```python
from build123d import *

# Parameters (mm, degrees)
F0_W     = 108.2
F0_H     = 88.2
F0_W_2   = 105
F0_H_2   = 85
F1_DEPTH = 80
F2_W     = 108.2
F2_H     = 88.2
F2_W_2   = 105
F2_H_2   = 85
F3_DEPTH = 2
F4_R     = 2


with BuildPart() as f1:
    # F0 (on Top) → F1 (new body)
    with BuildSketch(Plane.XY):
        with Locations((52.5, 42.5)):
            Rectangle(F0_W, F0_H)
        with Locations((52.5, 42.5)):
            Rectangle(F0_W_2, F0_H_2, mode=Mode.SUBTRACT)
    extrude(amount=F1_DEPTH)

    # F2 (on face) → F3 (join)
    with BuildSketch(Plane(origin=(0, 0, 0), x_dir=(1, 0, 0), z_dir=(0, 0, -1))):
        with Locations((52.5, -42.5)):
            Rectangle(F2_W, F2_H)
        with Locations((52.5, -42.5)):
            Rectangle(F2_W_2, F2_H_2, mode=Mode.SUBTRACT)
        with Locations((52.5, -42.5)):
            Rectangle(F2_W_2, F2_H_2)
    extrude(amount=F3_DEPTH)

    # F4
    f4_edges = [f1.edges().sort_by_distance(p)[0] for p in [
        (0, 85, 40),
        (105, 85, 40),
        (52.5, 0, 0),
        (0, 0, 40),
        (0, 42.5, 0),
        (52.5, 85, 0),
        (105, 42.5, 0),
        (105, 0, 40),
    ]]
    fillet(f4_edges, radius=F4_R)


solid = f1.part
```
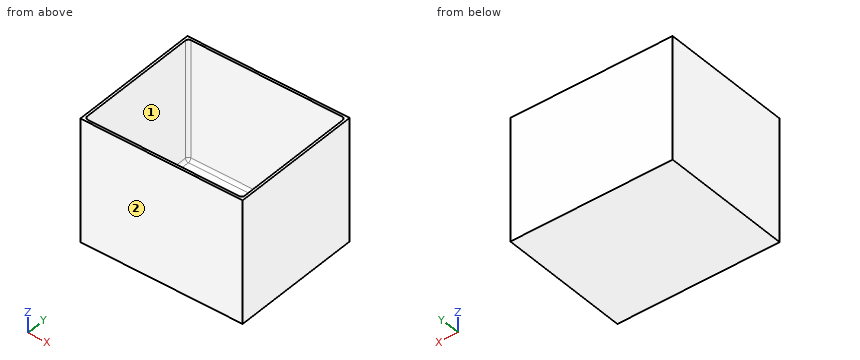
Check sheet for the modelled part. Datum: model origin and axes. Units: mm. Face numbers are marked on the shaded views. A direction names the side the tool comes from. Round coordinates to 2 decimals unless told otherwise and drop trailing zeros. Loops run counter-clockwise (first coordinate to the right, second up) from the corner with the lowest first, then second, coordinate; pieces in that order, holes last. Notation, with made-up numbers: (64.25, 79) -> (114.25, 79) arc R20 ccw to (114.25, 84) -> close; hole circle Ø6 at (36, 10). An arc over 180 degrees is marked (long way). Write item = value, one per line. Start each with the question number.
1) Set-up check for the marked faces 1 and 2: record each of +Z, -Z, +X, -X, +Y, -Y from which the full face is reachable in a straight line by a thin tool's end or side.
2) Thickness scan on probe 1 along Y at (x, z) = (28, 30); probe 2 along X at (y, z) = (48, 61.5); probe 3 along Z at (x, y) = (42.5, 55.5). Record the ranges inside material, lowest first.
3) Gauge pin test, flat end, axial feed: pin 1 Ø6 at (x, y) = (65.5, 19.5) entering from +Z. Record the tip position at first contact, or that the pin passes through.
4) Sectioned sample at B-B, the plane z = 57. Record the cut outline in (x, y).
5) Sectioned sample at C-C, the plane x = 63.5. Record the cut outline in (y, z).
6) Sectioned sample at A-A, the plane y = 70.5. Record the cut outline in (x, z), plus the area to 3 significant figures.
Results are:
q1.face_1 = +Z
q1.face_2 = +Z, -Z, +X, -X, -Y
q2.probe_1 = -1.6 to 0, 85 to 86.6
q2.probe_2 = -1.6 to 0, 105 to 106.6
q2.probe_3 = -2 to 0
q3.pin_1 = 0
q4.outline = (-1.6, -1.6) -> (106.6, -1.6) -> (106.6, 86.6) -> (-1.6, 86.6) -> close; hole (0, 2) arc R2 ccw to (2, 0) -> (103, 0) arc R2 ccw to (105, 2) -> (105, 83) arc R2 ccw to (103, 85) -> (2, 85) arc R2 ccw to (0, 83) -> close
q5.outline = (-1.6, -2) -> (86.6, -2) -> (86.6, 80) -> (85, 80) -> (85, 2) arc R2 cw to (83, 0) -> (2, 0) arc R2 cw to (0, 2) -> (0, 80) -> (-1.6, 80) -> close
q6.outline = (-1.6, -2) -> (106.6, -2) -> (106.6, 80) -> (105, 80) -> (105, 2) arc R2 cw to (103, 0) -> (2, 0) arc R2 cw to (0, 2) -> (0, 80) -> (-1.6, 80) -> close
q6.area = 474 mm^2
